Autodesk Inventor part; units mm, degrees
ref_plane "YZ Plane" through (0, 0, 0) normal (1, 0, 0) x (0, 1, 0)
ref_plane "XZ Plane" through (0, 0, 0) normal (0, 1, 0) x (-1, 0, 0)
ref_plane "XY Plane" through (0, 0, 0) normal (0, 0, 1) x (1, 0, 0)
sketch "Sketch1" plane through (0, 0, 0) normal (0, 0, 1) x (1, 0, 0)
  circle A0 centre (0, 0) radius 9
  line L0 (-0.75, 10) -> (0.75, 10)
  line L1 (0.75, 10) -> (0.75, 0)
  line L2 (0.75, 0) -> (-0.75, 0)
  line L3 (-0.75, 0) -> (-0.75, 10)
  point P0 (-0.75, 8.9687)
  point P1 (0.75, 8.9687)
  dimension "d0" = 18
  dimension "d26" = 0.75
  dimension "d28" = 0
  dimension "d29" = 10
extrude "Extrusion1" add sketch "Sketch1" along normal blind 15.5 contours A0 L3 L2 L1 | L1 L2 L3 A0
sketch "Sketch2" plane through (0, 0, 0) normal (0, 0, -1) x (-1, 0, 0)
  line L0 (-1.5, -2.5) -> (1.5, -2.5)
  line L1 (1.5, -2.5) -> (1.5, 2.5)
  line L2 (1.5, 2.5) -> (-1.5, 2.5)
  line L3 (-1.5, 2.5) -> (-1.5, -2.5)
  point P0 (0, 0)
  dimension "d3" = 3
  dimension "d4" = 5
  dimension "d5" = 2.5
  dimension "d6" = 1.5
extrude "Extrusion2" cut sketch "Sketch2" against normal blind 10
sketch "Sketch3" plane through (0, 0, 15.5) normal (0, 0, 1) x (1, 0, 0)
  circle A0 centre (0, 0) radius 1.6
  dimension "d9" = 3.2
extrude "Extrusion3" [suppressed]
sketch "Sketch4" plane through (0, 0, 0) normal (0, 0, -1) x (-1, 0, 0)
  circle A0 centre (0, 0) radius 4.5
  dimension "d12" = 9
extrude "Extrusion4" [suppressed]
sketch "Sketch10" plane through (0, 0, 15.5) normal (0, 0, 1) x (1, 0, 0)
  line L0 (2.9589, 5.125) -> (5.9178, 0)
  line L1 (5.9178, 0) -> (2.9589, -5.125)
  line L2 (2.9589, -5.125) -> (-2.9589, -5.125)
  line L3 (-2.9589, -5.125) -> (-5.9178, 0)
  line L4 (-5.9178, 0) -> (-2.9589, 5.125)
  line L5 (-2.9589, 5.125) -> (2.9589, 5.125)
  point P0 (0, 0)
  point P1 (0, 0)
  dimension "d145" = 10.25
extrude "Extrusion7" cut sketch "Sketch10" against normal blind 8.3
ref_plane "Work Plane3" through (0, -9, 0) normal (0, -1, 0) x (1, 0, 0)
sketch "Sketch11" plane through (0, -9, 0) normal (0, -1, 0) x (1, 0, 0)
  circle A0 centre (-1.4401, 13) radius 1.45
  line L0 (9, 15.5) -> (-9, 15.5)
  point P0 (0, 0)
  dimension "d66" = 2.9
  dimension "d144" = 2.5
extrude "Extrusion8" cut sketch "Sketch11" against normal through all both and the other way through all
ref_plane "Work Plane4" through (-10.5, -2.5, 0) normal (-1, 0, 0) x (0, 0, 1)
sketch "Sketch12" plane through (-10.5, -2.5, 0) normal (-1, 0, 0) x (0, 0, 1)
  circle A0 centre (3.5, 2.5) radius 1.45
  point P0 (0, 2.5)
  dimension "d71" = 2.9
  dimension "d74" = 3.5
extrude "Extrusion9" cut sketch "Sketch12" against normal blind 22
sketch "Sketch13" plane through (0, 0, 0) normal (0, 0, -1) x (-1, 0, 0)
  circle A0 centre (0, 0) radius 9.25
  circle A1 centre (0, 0) radius 4.75
  dimension "d75" = 9.5
  dimension "d78" = 18.5
extrude "Extrusion10" [suppressed]
sketch "Sketch14" plane through (0, 0, -3.7) normal (0, 0, -1) x (-1, 0, 0)
  line L0 (-8, -5) -> (-10, -5)
  line L1 (-10, -5) -> (-10, 5)
  line L2 (-10, 5) -> (-8, 5)
  line L3 (-8, 5) -> (-8, -5)
  line L4 (10, -5) -> (8, -5)
  line L5 (8, -5) -> (8, 5)
  line L6 (8, 5) -> (10, 5)
  line L7 (10, 5) -> (10, -5)
  line L8 (8, 8) -> (-8, 8)
  line L9 (-8, 8) -> (-8, 10)
  line L10 (-8, 10) -> (8, 10)
  line L11 (8, 10) -> (8, 8)
  line L12 (8, -10) -> (-5, -10)
  line L13 (-5, -10) -> (-5, -8)
  line L14 (-5, -8) -> (8, -8)
  line L15 (8, -8) -> (8, -10)
  point P0 (0, 0)
  dimension "d79" = 8
  dimension "d80" = 2
  dimension "d81" = 5
  dimension "d82" = 5
  dimension "d83" = 8
  dimension "d84" = 2
  dimension "d85" = 5
  dimension "d86" = 5
  dimension "d89" = 8
  dimension "d90" = 8
  dimension "d91" = 2
  dimension "d92" = 2
  dimension "d93" = 8
  dimension "d94" = 8
  dimension "d95" = 8
  dimension "d96" = 5
extrude "Extrusion11" [suppressed]
sketch "Sketch15" plane through (0, 0, 0) normal (0, 0, -1) x (-1, 0, 0)
  line L0 (10, -10.5) -> (7, -10.5)
  line L1 (7, -10.5) -> (7, 10.5)
  line L2 (7, 10.5) -> (10, 10.5)
  line L3 (10, 10.5) -> (10, -10.5)
  line L4 (-10, -10.5) -> (-7, -10.5)
  line L5 (-7, -10.5) -> (-7, 10.5)
  line L6 (-7, 10.5) -> (-10, 10.5)
  line L7 (-10, 10.5) -> (-10, -10.5)
  line L8 (-9.5, 10.5) -> (9.5, 10.5)
  line L9 (9.5, 10.5) -> (9.5, 7)
  line L10 (9.5, 7) -> (-9.5, 7)
  line L11 (-9.5, 7) -> (-9.5, 10.5)
  line L12 (-1.5, 2.5) -> (1.5, 2.5)
  line L13 (-1.5, -2.5) -> (-1.5, 2.5)
  line L14 (1.5, 2.5) -> (1.5, -2.5)
  line L15 (1.5, -2.5) -> (-1.5, -2.5)
  line L16 (-9.5, -7) -> (9.5, -7)
  line L17 (9.5, -7) -> (9.5, -10.5)
  line L18 (9.5, -10.5) -> (-9.5, -10.5)
  line L19 (-9.5, -10.5) -> (-9.5, -7)
  point P0 (0, 0)
  point P1 (-7, 7)
  point P2 (7, 7)
  point P3 (7, -7)
  point P4 (-7, -7)
  dimension "d101" = 8
  dimension "d102" = 8
  dimension "d103" = 8
  dimension "d106" = 8
  dimension "d107" = 8
  dimension "d109" = 8
  dimension "d110" = 8
  dimension "d111" = 8
  dimension "d113" = 8
  dimension "d114" = 8
  dimension "d115" = 3
  dimension "d118" = 7
  dimension "d119" = 7
  dimension "d120" = 7
  dimension "d121" = 7
  dimension "d146" = 3
extrude "Extrusion12" cut sketch "Sketch15" against normal blind 16.25 contours L0 L17 L16 L1 L10 L9 L2 L3 | L0 L1 L16 L17 | L18 L5 L16 L1 | L9 L10 L1 L2 | L4 L19 L16 L5 | L1 L10 L5 L8 | L16 L19 L4 L7 L6 L11 L10 L5 | L5 L10 L11 L6
sketch "Sketch17" plane through (0, 0, 0) normal (0, 0, -1) x (-1, 0, 0)
  line L0 (4.5, 4.5) -> (7, 4.5)
  line L1 (7, 4.5) -> (7, 7)
  line L2 (7, 7) -> (4.5, 7)
  line L3 (4.5, 7) -> (4.5, 4.5)
  line L4 (5.6569, 7) -> (-5.6569, 7)
  line L5 (7, -5.6569) -> (7, 5.6569)
  line L6 (7, -7) -> (4.5, -7)
  line L7 (4.5, -7) -> (4.5, -4.5)
  line L8 (4.5, -4.5) -> (7, -4.5)
  line L9 (7, -4.5) -> (7, -7)
  line L10 (-7, -7) -> (-4.5, -7)
  line L11 (-4.5, -7) -> (-4.5, -4.5)
  line L12 (-4.5, -4.5) -> (-7, -4.5)
  line L13 (-7, -4.5) -> (-7, -7)
  line L14 (-4.5, 7) -> (-7, 7)
  line L15 (-7, 7) -> (-7, 4.5)
  line L16 (-7, 4.5) -> (-4.5, 4.5)
  line L17 (-4.5, 4.5) -> (-4.5, 7)
  line L18 (-5.6569, -7) -> (5.6569, -7)
  line L19 (-7, 5.6569) -> (-7, -5.6569)
  point P0 (0, 0)
  point P1 (7, -4.5)
  point P2 (-4.5, 7)
  dimension "d128" = 2.5
  dimension "d129" = 2.5
  dimension "d130" = 2.5
  dimension "d131" = 2.5
  dimension "d132" = 2.5
  dimension "d133" = 2.5
  dimension "d134" = 2.5
  dimension "d135" = 2.5
extrude "Extrusion14" [suppressed]
sketch "Sketch18" plane through (0, 0, 0) normal (0, 0, -1) x (-1, 0, 0)
  circle A0 centre (0, 0) radius 10.5
  line L0 (-1.5, -2.5) -> (-1.5, 2.5)
  line L1 (1.5, 2.5) -> (1.5, -2.5)
  line L2 (-1.5, 2.5) -> (1.5, 2.5)
  line L3 (1.5, 2.5) -> (1.5, -2.5)
  line L4 (1.5, -2.5) -> (-1.5, -2.5)
  line L5 (-1.5, -2.5) -> (-1.5, 2.5)
  dimension "d138" = 21
extrude "Extrusion15" add sketch "Sketch18" along normal blind 3
chamfer "Chamfer1" distance 5 angle 45 4 edges at (-1.5, 0, -3) (1.5, 0, -3) (0, 2.5, -3) (0, -2.5, -3)
equation "\"d84\" = d80"
equation "\"d91\" = d80"
equation "\"d92\" = d80"
equation "\"d128\" = d129"
equation "\"d130\" = d129"
equation "\"d131\" = d129"
equation "\"d132\" = d129"
equation "\"d133\" = d129"
equation "\"d134\" = d129"
equation "\"d135\" = d129"
properties part number "6mm_shaft_couple_sideclip_v2"
Design review of the part built by this model. Coordinates are the model's own, in mm. A direction names the side the tool comes from. Round coordinates to 2 decimals unless told otherwise and drop trailing zeros. Write each loop counter-clockwise with the first axis right and the second up, starting at its lowest first coordinate (ties: lowest second). Pieces come first, ordered by that corner, then holes. Notation, with made-up numbers: (84, 19.25) -> (122, 19.25) arc R12 cw to (122, 32.25) -> close; hole circle Ø10 at (77.5, -38.75). An arc over 180 degrees is marked (long way). One line per item, written item: value. Start each with the question number.
Q1. The part is to be moulded in two halves that separate along X. For faces 6 (the face through (-10, -3.2, -1.5)), 7 (the face through (4.5, -0.1, -1)), 8 (the face through (-6.355, -6.373, 7.642)), 9 (the face through (7, 0, 8)), say which applies: pulls with the +X half, pulls with the -X half, needs draft (parallel to the pull), parting line crosses it, or undercut.
Q2. Add section B-B (z = 11). Give the boundary of the cut face in (x, y) (3 decimals).
Q3. Insertion check: P1, Ø6.5, axis at x = -1, z = 10, coming from the -Y side; P2, Ø4.5, axis at y = 0, z = 3.5, coming from the -X side; P3, Ø3, axis at x = 4, y = 1, coming from the -Z side; P4, Ø2.5, axis at x = -1.44, z = 13, coming from the -Y side. Each pin has a flat end and moves straight along its axis. Give the tip position at first contact, or say it passes through.
Q4. To check wall thickness, follow probe 1 along Y at (x, z) = (0.25, 11) (3 decimals); probe 2 along Y at (x, z) = (3.85, 3.5); probe 3 along Y at (x, z) = (4.75, 2). State the ranges of each line that lie inside material, in increasing order.
Q5. Add section C-C (x = 0.75). Give the boundary of the cut face in (y, z) (3 decimals).
Q6. Tool access review of faces 1 (the face through (0, 2.5, 5)), 2 (the face through (0, -5.125, 11)), 3 (the face through (6.373, -6.355, 7.642)), 4 (the face through (0, 7, 8)), 5 (the face through (-0.1, -5.5, -1)): name each direction out of +Z, -Z, +X, -X, +Y, -Y from which nothing blocks a thin tool from reaching the whole face with its end or side.
Q7. Add section D-D (z = 13). Give the boundary of the cut face in (x, y) (3 decimals).
Q8. Add section A-A (z = 3.5). Give the boundary of the cut face in (x, y).
Response:
1. face 6: parting line crosses it
1. face 7: undercut
1. face 8: pulls with the -X half
1. face 9: pulls with the +X half
2. outline: (-7, -5.657) arc R9 ccw to (-5.657, -7) -> (5.657, -7) arc R9 ccw to (7, -5.657) -> (7, 5.657) arc R9 ccw to (5.657, 7) -> (-5.657, 7) arc R9 ccw to (-7, 5.657) -> close; hole (-5.918, 0) -> (-2.959, -5.125) -> (2.959, -5.125) -> (5.918, 0) -> (2.959, 5.125) -> (-2.959, 5.125) -> close
3. P1: stops at y = -7
3. P2: stops at x = -7
3. P3: stops at z = -2
3. P4: passes through
4. probe 1: y = -7 to -5.125, 5.125 to 7
4. probe 2: y = -7 to -1.45, 1.45 to 7
4. probe 3: y = -7 to 7
5. outline: (-10.473, -3) -> (-7.5, -3) -> (-2.5, 2) -> (-2.5, 7.2) -> (-5.125, 7.2) -> (-5.125, 15.5) -> (-7, 15.5) -> (-7, 0) -> (-10.473, 0) -> close; (2.5, 2) -> (7.5, -3) -> (10.473, -3) -> (10.473, 0) -> (7, 0) -> (7, 15.5) -> (5.125, 15.5) -> (5.125, 7.2) -> (2.5, 7.2) -> close
6. face 1: +Z, -Z
6. face 2: +Z
6. face 3: +Z, +X, -Y
6. face 4: +Z, +X, -X, +Y
6. face 5: -Z
7. outline: (-7, -5.657) arc R9 ccw to (-5.657, -7) -> (-2.89, -7) -> (-2.89, -5.125) -> (-2.959, -5.125) -> (-5.918, 0) -> (-2.959, 5.125) -> (-2.89, 5.125) -> (-2.89, 7) -> (-5.657, 7) arc R9 ccw to (-7, 5.657) -> close; (0.01, -7) -> (5.657, -7) arc R9 ccw to (7, -5.657) -> (7, 5.657) arc R9 ccw to (5.657, 7) -> (0.01, 7) -> (0.01, 5.125) -> (2.959, 5.125) -> (5.918, 0) -> (2.959, -5.125) -> (0.01, -5.125) -> close
8. outline: (-7, -5.66) arc R9 ccw to (-5.66, -7) -> (5.66, -7) arc R9 ccw to (7, -5.66) -> (7, -1.45) -> (1.5, -1.45) -> (1.5, -2.5) -> (-1.5, -2.5) -> (-1.5, -1.45) -> (-7, -1.45) -> close; (-7, 1.45) -> (-1.5, 1.45) -> (-1.5, 2.5) -> (1.5, 2.5) -> (1.5, 1.45) -> (7, 1.45) -> (7, 5.66) arc R9 ccw to (5.66, 7) -> (-5.66, 7) arc R9 ccw to (-7, 5.66) -> close
